Geometry check sheet. Reference: drawing and pictorial views, mm from the part's lowest x, y, z. A direction names the side the tool comes from. Round coordinates to 2 decimals unless told otherwise and drop trailing zeros. Order: outer loops, then holes, each group sorted by start corner. A loop starts at its lowest first (then second) coordinate and runs counter-clockwise, first axis right, second up.
(1) Material ranges on line 1 along Y through (x, z) = (43, 13.5); line 2 along Y through (x, z) = (27.5, 28); line 3 along Y through (x, z) = (91, 20), recorded low to high.
(2) Sectioned sample at A-A (z = 25). Record the boundary of the cut face in (x, y) (1 decimal).
(3) Sectioned sample at C-C (x = 90.5). Record the boundary of the cut face in (y, z).
(4) Sectioned sample at D-D (z = 13.5). Record the boundary of the cut face in (x, y) (1 decimal), plus the area to 3 significant figures.
(5) Go/stop test with flat-tipped pins: pin 1 (5 mm diameter, centred on x = 48.5, z = 30, fed in from +Y); pin 2 (1 mm diameter, centred on y = 77, z = 17, fed in from +X); pin 3 (2 mm diameter, centred on y = 82, z = 39.5, fed in from -X). Record where each tip stops, or that it passes through.
(6) Set-up check for the marked faces 4, 5 and 6: record each of +Z, -Z, +X, -X, +Y, -Y from which the full face is reachable in a straight line by a thin tool's end or side.
(7) Sectioned sample at B-B (x = 48). Record the boundary of the cut face in (y, z).
(8) Release check for a two-part mould opening along Z. For the marked faces 1, 2 and 3 record: +Z half, -Z half, draft (parallel to the pull), parting line (faces both ways), or undercut.
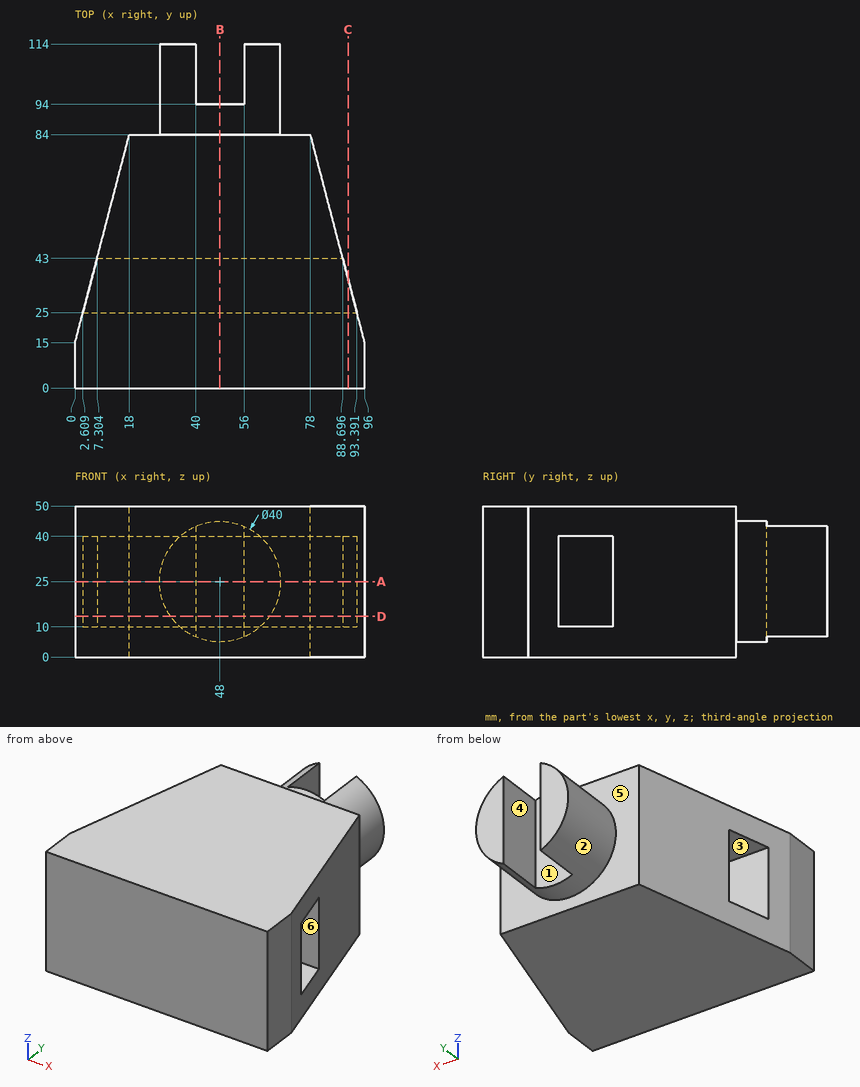
Answer below:
1. line 1: y = 0 to 25, 43 to 94
1. line 2: y = 0 to 25, 43 to 84
1. line 3: y = 0 to 25
2. outline: (0, 0) - (96, 0) - (96, 15) - (93.4, 25) - (2.6, 25) - (0, 15) - close; (7.3, 43) - (88.7, 43) - (78, 84) - (68, 84) - (68, 114) - (56, 114) - (56, 94) - (40, 94) - (40, 114) - (28, 114) - (28, 84) - (18, 84) - close
3. outline: (0, 0) - (36.08, 0) - (36.08, 10) - (25, 10) - (25, 40) - (36.08, 40) - (36.08, 50) - (0, 50) - close
4. outline: (0, 0) - (96, 0) - (96, 15) - (93.4, 25) - (2.6, 25) - (0, 15) - close; (7.3, 43) - (88.7, 43) - (78, 84) - (64.4, 84) - (64.4, 114) - (56, 114) - (56, 94) - (40, 94) - (40, 114) - (31.6, 114) - (31.6, 84) - (18, 84) - close
4. area: 5,930 mm2
5. pin 1: stops at y = 94
5. pin 2: stops at x = 79.96
5. pin 3: stops at x = 17.22
6. face 4: +Z, -Z, +Y
6. face 5: +Y
6. face 6: +X, -X
7. outline: (0, 0) - (84, 0) - (84, 5) - (94, 5) - (94, 45) - (84, 45) - (84, 50) - (0, 50) - close; hole (25, 10) - (43, 10) - (43, 40) - (25, 40) - close
8. face 1: draft
8. face 2: parting line
8. face 3: undercut
